For this review, take the finished solid that the model builds, in its own axes (mm). A direction names the side the tool comes from. Coordinates: 2 decimals unless noted, no trailing zeros. Order: outer loops, then holes, each group sorted by start corner. A loop starts at its lowest first (then second) coordinate and runs counter-clockwise, first axis right, second up. Notation, with made-up numbers: (21, -29) - (72, -29) arc R17 cw to (72, -8) - close; hole circle Ø8 at (78, 54.5). An arc over 180 degrees is marked (long way). One line per item, written item: value. Start each with the question number.
(1) Mouldability with a two-part tool opening along X and no side actions: class faces 4 (the flat face through (10, 2, 0)), 5 (the flat face through (-72, 2, -32.249)), 6 (the flat face through (-85.45, 2.46, -84.45)) as released by +X, released by -X, zero draft, split by the parting line, or undercut.
(2) Clearance check with flat-ended pins moving along their axes: pin 1 (1.5 mm diameter, centred on x = -77.5, y = 1.5, fed in from +Z); pin 2 (2.5 mm diameter, centred on x = -50.5, y = 3.5, fed in from -Z); pin 3 (2.5 mm diameter, centred on x = -119.5, y = 3, fed in from -Z); pin 4 (1.5 mm diameter, centred on y = 1.5, z = 60, fed in from -X). State where each tip first meets the part, or that it passes through.
(3) Consider section A-A on z = -81. Write out the cut boundary in (x, y), then the cut area to 3 significant figures.
(4) Consider section D-D on x = -24. Write out the cut boundary in (y, z).
(5) Consider section B-B on x = -80. Write out the cut boundary in (y, z), then the cut area to 3 significant figures.
(6) To check wall thickness, follow line 1 along Z through (x, y) = (-80, 0.3); line 2 along Z through (x, y) = (-55, 0.9); line 3 along Z through (x, y) = (-103, 2.55). State the ranges of each line that lie inside material, in increasing order.
(7) For faces 1 (the flat face through (-43.71, 2.465, 40.326)), 2 (the flat face through (5, 2, -5)), 3 (the flat face through (-72, 2, 32.249)), list the 3-axis set-ups (+Z, -Z, +X, -X, +Y, -Y) from which the entire face can be reached by the end or side of a thin tool; tool diameter is ignored.
Autodesk Inventor part; units mm, degrees
ref_plane "YZ Plane" through (0, 0, 0) normal (1, 0, 0) x (0, 1, 0)
ref_plane "XZ Plane" through (0, 0, 0) normal (0, 1, 0) x (-1, 0, 0)
ref_plane "XY Plane" through (0, 0, 0) normal (0, 0, 1) x (1, 0, 0)
sketch "Sketch1" plane through (0, 0, 0) normal (0, 1, 0) x (-1, 0, 0)
  line L0 (0, 0) -> (10, 0) construction
  line L1 (-10, 0) -> (-10, 5)
  line L2 (-10, 5) -> (0, 5)
  line L3 (-10, 0) -> (-10, -5)
  line L4 (-10, 0) -> (-5, 0) construction
  line L5 (-10, -5) -> (0, -5)
  line L6 (0, -5) -> (21.1309, -50.3154)
  line L7 (21.1309, -50.3154) -> (8.4524, -77.5046)
  line L8 (8.4524, -77.5046) -> (62.8308, -52.1475)
  line L9 (62.8308, -52.1475) -> (108.7169, -117.6797)
  line L10 (108.7169, -117.6797) -> (118.7169, -117.6797)
  line L11 (118.7169, -117.6797) -> (70.3694, -48.6322)
  line L12 (70.3694, -48.6322) -> (85.3694, -48.6322)
  line L13 (85.3694, -48.6322) -> (114.0482, -89.5898)
  line L14 (114.0482, -89.5898) -> (124.0482, -89.5898)
  line L15 (124.0482, -89.5898) -> (83.8979, -32.2492)
  line L16 (83.8979, -32.2492) -> (58.8979, -32.2492)
  line L17 (58.8979, -32.2492) -> (28.0903, -48.6322)
  line L18 (28.0903, -48.6322) -> (7.7442, -5)
  line L19 (7.7442, -5) -> (113.7169, -5)
  line L20 (113.7169, -5) -> (124.0482, 0)
  line L21 (-10, 0) -> (-10, 5)
  line L22 (-10, 5) -> (0, 5)
  line L23 (0, 5) -> (21.1309, 50.3154)
  line L24 (21.1309, 50.3154) -> (8.4524, 77.5046)
  line L25 (8.4524, 77.5046) -> (62.8308, 52.1475)
  line L26 (62.8308, 52.1475) -> (108.7169, 117.6797)
  line L27 (108.7169, 117.6797) -> (118.7169, 117.6797)
  line L28 (118.7169, 117.6797) -> (70.3694, 48.6322)
  line L29 (70.3694, 48.6322) -> (85.3694, 48.6322)
  line L30 (85.3694, 48.6322) -> (114.0482, 89.5898)
  line L31 (114.0482, 89.5898) -> (124.0482, 89.5898)
  line L32 (124.0482, 89.5898) -> (83.8979, 32.2492)
  line L33 (83.8979, 32.2492) -> (58.8979, 32.2492)
  line L34 (58.8979, 32.2492) -> (28.0903, 48.6322)
  line L35 (28.0903, 48.6322) -> (7.7442, 5)
  line L36 (7.7442, 5) -> (113.7169, 5)
  line L37 (113.7169, 5) -> (124.0482, 0)
  dimension "d2" = 5
  dimension "d4" = 10
  dimension "d6" = 5
  dimension "d7" = 90
  dimension "d8" = 10
  dimension "d9" = 90
  dimension "d10" = 50
  dimension "d12" = 30
  dimension "d13" = 130
  dimension "d14" = 60
  dimension "d15" = 80
  dimension "d16" = 100
  dimension "d17" = 10
  dimension "d18" = 125
  dimension "d19" = 15
  dimension "d20" = 55
  dimension "d21" = 50
  dimension "d22" = 125
  dimension "d23" = 10
  dimension "d24" = 125
  dimension "d25" = 70
  dimension "d26" = 55
extrude "Extrusion1" add sketch "Sketch1" along normal blind 5
properties part number "QQI"
Geometry check:
1. face 4: released by +X
1. face 5: zero draft
1. face 6: undercut
2. pin 1: stops at z = 74.17
2. pin 2: stops at z = -58.48
2. pin 3: stops at z = -117.68
2. pin 4: stops at x = -103.85
3. outline: (-118.03, 0) - (-108.03, 0) - (-108.03, 5) - (-118.03, 5) - close; (-93.03, 0) - (-83.03, 0) - (-83.03, 5) - (-93.03, 5) - close
3. area: 100 mm^2
4. outline: (0, -70.25) - (5, -70.25) - (5, -39.86) - (0, -39.86) - close; (0, -5) - (5, -5) - (5, 5) - (0, 5) - close; (0, 39.86) - (5, 39.86) - (5, 70.25) - (0, 70.25) - close
5. outline: (0, -76.67) - (5, -76.67) - (5, -62.39) - (0, -62.39) - close; (0, -48.63) - (5, -48.63) - (5, -32.25) - (0, -32.25) - close; (0, -5) - (5, -5) - (5, 5) - (0, 5) - close; (0, 32.25) - (5, 32.25) - (5, 48.63) - (0, 48.63) - close; (0, 62.39) - (5, 62.39) - (5, 76.67) - (0, 76.67) - close
5. area: 357 mm^2
6. line 1: z = -76.67 to -62.39, -48.63 to -32.25, -5 to 5, 32.25 to 48.63, 62.39 to 76.67
6. line 2: z = -55.8 to -34.32, -5 to 5, 34.32 to 55.8
6. line 3: z = -109.52 to -95.23, -73.81 to -59.53, -5 to 5, 59.53 to 73.81, 95.23 to 109.52
7. face 1: +Y, -Y
7. face 2: -Z, +X, +Y, -Y
7. face 3: -X, +Y, -Y
